Geometry check sheet. Reference: the model listing, model coordinates, mm. Face numbers are marked on the shaded views. Give positions to 0.01 mm unless a question says otherwise; leave off trailing zeros. Write each loop counter-clockwise with the first axis right and the second up, starting at its lowest first coordinate (ties: lowest second). Pieces come first, ordered by that corner, then holes. Notation, with made-up numbers: (65.25, 40) -> (71.25, 40) arc R10 ccw to (71.25, 50) -> close; hole circle Ø3 at (-37.75, 15.5). An arc over 180 degrees is marked (long way). One line per item, written item: value.
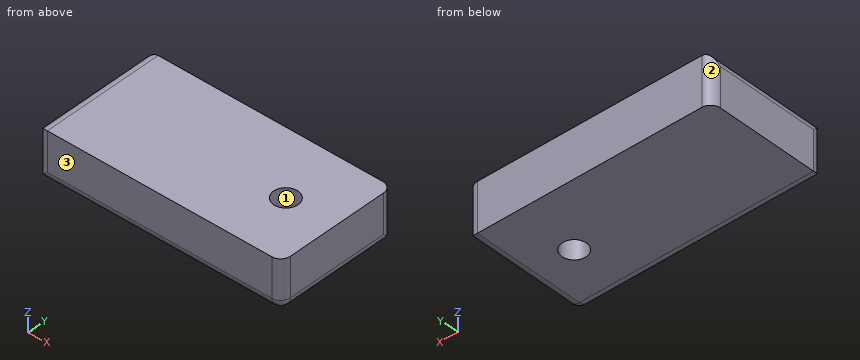
from build123d import *

# Parameters (mm, degrees)
F0_W           = 127
F0_H           = 63.5
F1_DEPTH       = 25.4
F3_D           = 12.7
F3_CBORE_D     = 12.7
F3_CBORE_DEPTH = 6.35
F4_R           = 5.08


with BuildPart() as f1:
    # F0 (on Top) → F1 (new body)
    with BuildSketch(Plane.XY):
        with Locations((63.5, 31.75)):
            Rectangle(F0_W, F0_H)
    extrude(amount=F1_DEPTH)

    # F3 (through all)
    with Locations(Plane(origin=(0, 0, 0), x_dir=(1, 0, 0), z_dir=(0, 0, -1))):
        with Locations((101.218447, -30.816942)):
            CounterBoreHole(F3_D / 2, F3_CBORE_D / 2, F3_CBORE_DEPTH)

    # F4
    f4_edges = [f1.edges().sort_by_distance(p)[0] for p in [
        (127, 31.75, 0),
        (127, 63.5, 12.7),
        (127, 0, 12.7),
        (63.5, 0, 0),
        (0, 0, 12.7),
        (0, 31.75, 25.4),
        (0, 63.5, 12.7),
    ]]
    fillet(f4_edges, radius=F4_R)


solid = f1.part
1) Sectioned sample at D-D on y = 26. Record the cut outline in (x, z), plus the area to 3 significant figures.
Verdict:
outline: (0, 0) -> (97.08, 0) -> (97.08, 25.4) -> (5.08, 25.4) arc R5.08 ccw to (0, 20.32) -> close; (105.36, 0) -> (121.92, 0) arc R5.08 ccw to (127, 5.08) -> (127, 25.4) -> (105.36, 25.4) -> close
area: 3,000 mm^2
2) Sectioned sample at B-B on x = 106. Record the cut outline in (y, z), plus the area to 3 significant figures.
Verdict:
outline: (0, 5.08) arc R5.08 ccw to (5.08, 0) -> (26.64, 0) -> (26.64, 25.4) -> (0, 25.4) -> close; (35, 0) -> (63.5, 0) -> (63.5, 25.4) -> (35, 25.4) -> close
area: 1,400 mm^2
3) Mould release check, pull along X, two halves, no side actions. Record for the marked faces 1, 2 and 3: released by +X, released by -X, zero draft, split by the parting line, or undercut.
Verdict:
face 1: undercut
face 2: released by -X
face 3: zero draft
4) Sectioned sample at C-C on z = 22. Record the cut outline in (x, y), plus the area to 3 significant figures.
Verdict:
outline: (0.29, 3.4) arc R5.08 ccw to (5.08, 0) -> (121.92, 0) arc R5.08 ccw to (127, 5.08) -> (127, 58.42) arc R5.08 ccw to (121.92, 63.5) -> (5.08, 63.5) arc R5.08 ccw to (0.29, 60.1) -> close; hole circle Ø12.7 at (101.22, 30.82)
area: 7,900 mm^2
5) Scan lines: probe 1 along X at (y, z) = (34, 5.75); probe 2 along X at (y, z) = (32, 1.75); probe 3 along X at (y, z) = (10.5, 20.5). Record each from-to range of solid material in increasing order.
Verdict:
probe 1: 0 to 95.72, 106.71 to 127
probe 2: 0 to 94.98, 107.46 to 125.76
probe 3: 0 to 127
6) Sectioned sample at A-A on y = 34.5. Record the cut outline in (x, z), plus the area to 3 significant figures.
Verdict:
outline: (0, 0) -> (96.05, 0) -> (96.05, 25.4) -> (5.08, 25.4) arc R5.08 ccw to (0, 20.32) -> close; (106.39, 0) -> (121.92, 0) arc R5.08 ccw to (127, 5.08) -> (127, 25.4) -> (106.39, 25.4) -> close
area: 2,950 mm^2
